from build123d import *

# Parameters (mm, degrees)
F0_W     = 20.2084705234
F0_H     = 20.1108679175
F1_DEPTH = 20
F3_R     = 3.9554921295
F3_R_2   = 2.3007028816
F3_R_3   = 1.330304551
F4_DEPTH = 25


with BuildPart() as f1:
    # F0 (on Top) → F1 (new body)
    with BuildSketch(Plane.XY):
        with Locations((-10.1042352617, -10.0554339588)):
            Rectangle(F0_W, F0_H)
    extrude(amount=F1_DEPTH)

    # F3 (on face) → F4 (cut)
    with BuildSketch(Plane(origin=(0, 0, 0), x_dir=(1, 0, 0), z_dir=(0, 0, -1))):
        with Locations((-8.2629937679, 10.3565575555)):
            Circle(F3_R)
        with Locations((-8.2629937679, 10.3565575555)):
            Circle(F3_R_2, mode=Mode.SUBTRACT)
        with Locations((-8.2629937679, 10.3565575555)):
            Circle(F3_R_2)
        with Locations((-8.2629937679, 10.3565575555)):
            Circle(F3_R_3, mode=Mode.SUBTRACT)
        with Locations((-8.2629937679, 10.3565575555)):
            Circle(F3_R_3)
    extrude(amount=-F4_DEPTH, mode=Mode.SUBTRACT)


solid = f1.part
Model file for the job. Use its own axes, mm. Give positions to 0.01 mm unless a question says otherwise; leave off trailing zeros. Loops run counter-clockwise (first coordinate to the right, second up) from the corner with the lowest first, then second, coordinate; pieces in that order, holes last. Notation, with made-up numbers: (-23, 77) -> (-6, 77) arc R14 cw to (-6, 90) -> close; hole circle Ø9 at (43, -13). An arc over 180 degrees is marked (long way). Use a Markdown table: item, result. Add a question column.
(1) Mould opens along X. For faces 1 (the flat face through (0, -10, 10)), 2 (the flat face through (-10, 0, 10)), 3 (the cylindrical face through (-6.438, -6.847, 9.86)), 4 (the flat face through (-20.208, -10, 10)) say: +X half, -X half, draft (parallel to the pull), parting line (faces both ways), or undercut.
(2) Wall check: line 1 along X through (y, z) = (-10.5, 17.25); line 2 along X through (y, z) = (-7.75, 12); line 3 along Y through (x, z) = (-9.75, 11.75). Give the ranges that are in metal, low to high.
(3) Slice it at B-B on x = -10. List the corners of the cut face in (y, z).
(4) Slice it at A-A on y = -8.25. List the corners of the cut face in (x, z), and give its area (3 significant figures).
(5) Slice it at C-C on z = 6. List the corners of the cut face in (x, y).
Filled sheet:
| question | item | result |
|---|---|---|
| 1 | face 1 | +X half |
| 1 | face 2 | draft |
| 1 | face 3 | undercut |
| 1 | face 4 | -X half |
| 2 | line 1 | -20.21 to -12.22, -4.31 to 0 |
| 2 | line 2 | -20.21 to -11.24, -5.29 to 0 |
| 2 | line 3 | -20.11 to -14.02, -6.69 to 0 |
| 3 | outline | (-20.11, 0) -> (-13.91, 0) -> (-13.91, 20) -> (-20.11, 20) -> close; (-6.8, 0) -> (0, 0) -> (0, 20) -> (-6.8, 20) -> close |
| 4 | outline | (-20.21, 0) -> (-11.61, 0) -> (-11.61, 20) -> (-20.21, 20) -> close; (-4.92, 0) -> (0, 0) -> (0, 20) -> (-4.92, 20) -> close |
| 4 | area | 270 mm2 |
| 5 | outline | (-20.21, -20.11) -> (0, -20.11) -> (0, 0) -> (-20.21, 0) -> close; hole circle Ø7.91 at (-8.26, -10.36) |
